Autodesk Inventor part; units mm, degrees
ref_plane "YZ Plane" through (0, 0, 0) normal (1, 0, 0) x (0, 1, 0)
ref_plane "XZ Plane" through (0, 0, 0) normal (0, 1, 0) x (-1, 0, 0)
ref_plane "XY Plane" through (0, 0, 0) normal (0, 0, 1) x (1, 0, 0)
sketch "Boceto1" plane through (0, 0, 0) normal (0, 1, 0) x (-1, 0, 0)
  line L0 (-15, 66) -> (-49, 66)
  line L1 (45, 18.438) -> (49, 18.438)
  line L2 (-49, 66) -> (49, 66)
  line L3 (49, 66) -> (49, 18.438)
  line L4 (49, 18.438) -> (-49, 18.438)
  line L5 (-49, 18.438) -> (-49, 66)
  line L6 (-47, 51) -> (-45, 51)
  line L7 (-47, 51) -> (-45, 51)
  line L8 (-45, 51) -> (-45, 31)
  line L9 (-45, 31) -> (-47, 31)
  line L10 (-47, 31) -> (-47, 51)
  line L11 (45, 51.5) -> (45, 42.5)
  line L12 (47, 51) -> (47, 31)
  line L13 (45, 51.5) -> (47, 51.5)
  line L14 (47, 51.5) -> (47, 31)
  line L15 (47, 31) -> (45, 31)
  line L16 (45, 31) -> (45, 51.5)
  point P0 (0, 0)
extrude "Extrusión1" add sketch "Boceto1" along normal blind 1.5 contours L2 L3 L1 L4 L5 L0 | L6 L8 L9 L10 | L13 L14 L12 L15 L16 L11
sketch "Boceto2" plane through (0, 0, 0) normal (0, -1, 0) x (1, 0, 0)
  line L0 (-47, 51) -> (-45, 51)
  line L1 (-45, 51) -> (-45, 30.9876)
  line L2 (-45, 30.9876) -> (-47, 30.9876)
  line L3 (-47, 30.9876) -> (-47, 51)
  line L4 (45, 51) -> (47, 51)
  line L5 (47, 51) -> (47, 31)
  line L6 (47, 31) -> (45, 31)
  line L7 (45, 31) -> (45, 51)
  point P0 (0, 0)
extrude "Extrusión2" add sketch "Boceto2" along normal blind 10
sketch "Boceto3" plane through (-47, 0, 30.9876) normal (-1, 0, 0) x (0, 0, 1)
  line L0 (0, -10) -> (20.0124, -10)
  line L1 (20.0124, 0) -> (20.0124, -10)
  line L2 (0, -10) -> (20.0124, -10)
  line L3 (20.0124, -10) -> (20.0124, -7)
  line L4 (20.0124, -7) -> (0, -7)
  line L5 (0, -7) -> (0, -10)
  dimension "d4" = 3
extrude "Extrusión3" add sketch "Boceto3" along normal blind 1
sketch "Boceto5" plane through (47, 0, 51) normal (1, 0, 0) x (0, 0, -1)
  line L0 (20.0124, -10) -> (0, -10)
  line L1 (0, -10) -> (20.0124, -10)
  line L2 (20.0124, -10) -> (20.0124, -7)
  line L3 (20.0124, -7) -> (0, -7)
  line L4 (0, -7) -> (0, -10)
  point P0 (51, 0)
  dimension "d8" = 3
extrude "Extrusión4" add sketch "Boceto5" along normal blind 1
sketch "Boceto7" plane through (-49, 0, 66) normal (0, 0, 1) x (1, 0, 0)
  line L0 (49, 0) -> (49, 1.3987)
  line L1 (4, -10) -> (1, -10)
  line L2 (2, -7) -> (1, -7)
  line L3 (4, -10) -> (1, -10)
  line L4 (1, -10) -> (1, -7)
  line L5 (4, -7) -> (4, -10)
  line L6 (1, -7) -> (4, -10)
  line L7 (1, -10) -> (4, -10)
  line L8 (1, -7) -> (1, -10)
  line L9 (94, -10) -> (97, -10)
  line L10 (97, -10) -> (97, -7)
  line L11 (97, -7) -> (94, -10)
extrude "Extrusión5" cut sketch "Boceto7" against normal blind 48.25
equation "\"Radio_pliegue\" = Grosor"
equation "\"Anchura_desahogo_plegado\" = Grosor"
equation "\"Profundidad_desahogo_plegado\" = 0.5 * Grosor"
equation "\"Tamaño_destalonado\" = 4 * Grosor"
equation "\"Remanente_mínimo\" = 2 * Grosor"
equation "\"Radiodetransición\" = Radio_pliegue"
equation "\"Tamaño_de_radio_de_Jacobi\" = Radio_pliegue"
equation "\"TamañoSeparación\" = Grosor"
properties part number "TapaOnixium"
Can you work these out from the model? Positions are in its coordinate system, mm. A direction names the side the tool comes from. Round coordinates to 2 decimals unless told otherwise and drop trailing zeros. Order: outer loops, then holes, each group sorted by start corner. A loop starts at its lowest first (then second) coordinate and runs counter-clockwise, first axis right, second up.
(1) We'd pull the mould along X, two halves only. Please class faces 4 (the face through (47, -3, 41)), 5 (the face through (-47, -8, 41)), 6 (the face through (-45, -5, 41)): +X half, -X half, draft (parallel to the pull), parting line (faces both ways), or undercut.
Results are:
face 4: +X half
face 5: -X half
face 6: undercut
(2) If we section it at B-B (z = 41.5): Please give me the cut outline in (x, y).
Results are:
outline: (-49, 0) - (-47, 0) - (-47, -7) - (-48, -7) - (-45, -10) - (-45, 0) - (45, 0) - (45, -10) - (48, -7) - (47, -7) - (47, 0) - (49, 0) - (49, 1.5) - (-49, 1.5) - close
(3) If we section it at D-D (z = 57.5): Please give me the cut outline in (x, y).
Results are:
outline: (-49, 0) - (49, 0) - (49, 1.5) - (-49, 1.5) - close
(4) On a 3-axis mill with a long thin cutter (end or side, diameter ignored), from which of +Z, -Z, +X, -X, +Y, -Y can I reach the whole of each face in a straight line? I mean faces 1 (the face through (-46, -5, 51)), 2 (the face through (45, -5, 41)), 3 (the face through (-47, -3, 41)). Say none if no direction works.
Results are:
face 1: +Z, +X, -X, -Y
face 2: +Z, -Z, -Y
face 3: +Z, -Z, -X
(5) If we section it at C-C (x = 22.5): Please give me the cut outline in (y, z).
Results are:
outline: (0, 18.44) - (1.5, 18.44) - (1.5, 66) - (0, 66) - close
(6) If I drill on L1, parallel to X at y = -6, z = 37; L2, parallel to Y at x = 18, z = 43; L3, parallel to X at y = -8.75, z = 39.5, over which ranges is the centre line in solid material (lowest first)?
Results are:
L1: x = -47 to -45, 45 to 47
L2: y = 0 to 1.5
L3: x = -46.25 to -45, 45 to 46.25
(7) I'm going to push flat-ended pins straight in: pin 1 (5.5 mm diameter, centred on y = -2.5, z = 45.5, fed in from -X); pin 2 (3 mm diameter, centred on x = -20, z = 32.5, fed in from -Y); pin 3 (0.9 mm diameter, centred on x = 46.5, y = -4, fed in from +Z); pin 4 (0.8 mm diameter, centred on x = 47.5, y = -7.5, fed in from -Z). Where does each tip first touch, or does it pass through?
Results are:
pin 1: stops at x = -49
pin 2: stops at y = 0
pin 3: stops at z = 51
pin 4: stops at z = 30.99
(8) If we section it at A-A (y = -4.25): Please give me the cut outline in (x, z), plus the area to 3 significant figures.
Results are:
outline: (-47, 30.99) - (-45, 30.99) - (-45, 51) - (-47, 51) - close; (45, 31) - (47, 31) - (47, 51) - (45, 51) - close
area: 80.0 mm2
